```python
from build123d import *

# Parameters (mm, degrees)
BOSS_EXTRUDE1_DEPTH   = 20
FILLET1_R             = 6.35
F_5_0MM_DOWEL_HOLE1_D = 5
F_5_0MM_DOWEL_HOLE2_D = 5


with BuildPart() as part:
    # Sketch1 → Boss-Extrude1 (new body)
    with BuildSketch(Plane.XY):
        Polygon((0, 0), (0, 50.8), (9.525, 50.8), (9.525, 9.525), (50.8, 9.525), (50.8, 0), align=None)
    extrude(amount=-BOSS_EXTRUDE1_DEPTH)

    # Fillet1
    fillet1_edges = [part.edges().sort_by_distance(p)[0] for p in [
        (9.525, 50.8, -10),
        (9.525, 9.525, -10),
        (50.8, 9.525, -10),
    ]]
    fillet(fillet1_edges, radius=FILLET1_R)

    # Ø5.0mm Dowel Hole1 (through all)
    with Locations(Plane(origin=(0, 0, 0), x_dir=(-1, 0, 0), z_dir=(0, -1, 0))):
        with Locations((-25.4, 10)):
            Hole(F_5_0MM_DOWEL_HOLE1_D / 2)

    # Ø5.0mm Dowel Hole2 (through all)
    with Locations(Plane.ZY):
        with Locations((-10, 38.1)):
            Hole(F_5_0MM_DOWEL_HOLE2_D / 2)


solid = part.part
```
The listing builds one solid part. Answer for the finished solid, in the listing's coordinates (mm). A direction names the side the tool comes from. Give positions to 0.01 mm unless a question says otherwise; leave off trailing zeros. Loops run counter-clockwise (first coordinate to the right, second up) from the corner with the lowest first, then second, coordinate; pieces in that order, holes last. Notation, with made-up numbers: M 27.5,85 L 56.5,85 A23 ccw 56.5,96 Z; hole C 11,25.25 d1. An arc over 180 degrees is marked long. One line per item, written item: value.
Q1. For faces 1 (the face through (0, 25, -10)), 2 (the face through (30, 9.525, -10)), determine the directions among +Z, -Z, +X, -X, +Y, -Y from which every point of the face is accessible in a straight line to the end or side of a thin tool.
Working result:
face 1: +Z, -Z, -X, +Y, -Y
face 2: +Z, -Z, +X, +Y
Q2. A cutting plane is placed at C-C on z = -3.75. Determine the outline of the cut face in (x, y) (3 decimals).
Working result:
outline: M 0,0 L 50.8,0 L 50.8,3.175 A6.35 ccw 44.45,9.525 L 15.875,9.525 A6.35 cw 9.525,15.875 L 9.525,44.45 A6.35 ccw 3.175,50.8 L 0,50.8 Z
Q3. Find the intervals of material crossed by line 1 (X direction, y = 2.5, z = -10); line 2 (Z direction, x = 25.4, y = 7.25); line 3 (Y direction, x = 2.75, z = -10), in increasing order. Write a range as from..to.
Working result:
line 1: x = 0..22.9, 27.9..50.8
line 2: z = -20..-12.5, -7.5..0
line 3: y = 0..35.6, 40.6..50.8
Q4. A cutting plane is placed at D-D on x = 27. Determine the outline of the cut face in (y, z) (3 decimals), then the cut area to 3 significant figures.
Working result:
outline: M 0,-20 L 9.525,-20 L 9.525,-11.921 L 0,-11.921 Z; M 0,-8.079 L 9.525,-8.079 L 9.525,0 L 0,0 Z
area: 154 mm^2
Q5. Flat-ended cylindrical pins translate along their axes: P1, Ø6, axis at x = 25.4, z = -10, coming from the +Y side (3 decimals); P2, Ø10, axis at x = 18.5, y = 32.5, coming from the -Z side; P3, Ø2, axis at y = 43.5, z = -5.5, coming from the +X side (3 decimals). Find the tip coordinate at first contact, or state that the pin passes through.
Working result:
P1: stops at y = 9.525
P2: passes through
P3: stops at x = 9.525
Q6. A cutting plane is placed at A-A on y = 38.1. Determine the outline of the cut face in (x, z) (3 decimals), then the cut area to 3 significant figures.
Working result:
outline: M 0,-20 L 9.525,-20 L 9.525,-12.5 L 0,-12.5 Z; M 0,-7.5 L 9.525,-7.5 L 9.525,0 L 0,0 Z
area: 143 mm^2
Q7. A cutting plane is placed at B-B on z = -10. Determine the outline of the cut face in (x, y) (3 decimals).
Working result:
outline: M 0,0 L 22.9,0 L 22.9,9.525 L 15.875,9.525 A6.35 cw 9.525,15.875 L 9.525,35.6 L 0,35.6 Z; M 0,40.6 L 9.525,40.6 L 9.525,44.45 A6.35 ccw 3.175,50.8 L 0,50.8 Z; M 27.9,0 L 50.8,0 L 50.8,3.175 A6.35 ccw 44.45,9.525 L 27.9,9.525 Z
Q8. Determine the mould class of faces 3 (the face through (14, 9, 0)), 4 (the face through (4.83, 35.66, -9.46)), 5 (the face through (2, 50.8, -10)) for opening direction Z: +Z half, -Z half, draft (parallel to the pull), parting line (faces both ways), or undercut.
Working result:
face 3: +Z half
face 4: undercut
face 5: draft
